from build123d import *

# Parameters (mm, degrees)
F0_R     = 3
F0_R_2   = 18
F0_R_3   = 9
F0_R_4   = 4.5
F1_DEPTH = 5


with BuildPart() as f1:
    # F0 (on Top) → F1 (new body)
    with BuildSketch(Plane.XY):
        Polygon((52.5, 54.183173), (-66, 54.183173), (-66, -68.816827), (-66, -94.316827), (-16.5, -94.316827), (-16.5, -68.816827), (52.5, -68.816827), align=None)
        Polygon((-61.5, -86.816827), (-61.5, -77.816827), (-52.5, -77.816827), (-45, -77.816827), (-36, -77.816827), (-30, -77.816827), (-21, -77.816827), (-21, -86.816827), (-30, -86.816827), (-36, -86.816827), (-45, -86.816827), (-52.5, -86.816827), align=None, mode=Mode.SUBTRACT)
        with Locations((-57, -59.816827)):
            Circle(F0_R, mode=Mode.SUBTRACT)
        with Locations((-33, -32.316827)):
            Circle(F0_R_2, mode=Mode.SUBTRACT)
        with Locations((43.5, -59.816827)):
            Circle(F0_R, mode=Mode.SUBTRACT)
        with Locations((6, -32.316827)):
            Circle(F0_R_3, mode=Mode.SUBTRACT)
        with Locations((31.5, -32.316827)):
            Circle(F0_R_3, mode=Mode.SUBTRACT)
        with Locations((-29.488925, 2.183173)):
            Circle(F0_R, mode=Mode.SUBTRACT)
        with BuildLine():
            Line((-51, 12.183173), (-51, 36.183173))
            Line((-51, 36.183173), (-27, 36.183173))
            ThreePointArc((-27, 36.183173), (-23.25, 32.433173), (-27, 28.683173))
            Line((-27, 28.683173), (-43.5, 28.683173))
            Line((-43.5, 28.683173), (-43.5, 12.183173))
            Line((-43.5, 12.183173), (-51, 12.183173))
        make_face(mode=Mode.SUBTRACT)
        with Locations((-57, 45.183173)):
            Circle(F0_R, mode=Mode.SUBTRACT)
        with BuildLine():
            Line((-6, -1.316827), (-6, 16.683173))
            ThreePointArc((-6, 16.683173), (0, 22.683173), (6, 16.683173))
            Line((6, 16.683173), (6, -1.316827))
            ThreePointArc((6, -1.316827), (0, -7.316827), (-6, -1.316827))
        make_face(mode=Mode.SUBTRACT)
        with Locations((24, 2.183173)):
            Circle(F0_R, mode=Mode.SUBTRACT)
        with Locations((37, 2.183173)):
            Circle(F0_R_4, mode=Mode.SUBTRACT)
        with Locations((43.5, 45.183173)):
            Circle(F0_R, mode=Mode.SUBTRACT)
    extrude(amount=F1_DEPTH)


solid = f1.part
Check sheet for the modelled part. Datum: model origin and axes. Units: mm. A direction names the side the tool comes from. Round coordinates to 2 decimals unless told otherwise and drop trailing zeros. Loops run counter-clockwise (first coordinate to the right, second up) from the corner with the lowest first, then second, coordinate; pieces in that order, holes last. Notation, with made-up numbers: M 52.25,56 L 98.25,56 A31 ccw 98.25,85 Z; hole C 31,29.5 d10. An arc over 180 degrees is marked long. One line per question, with ' | ' between items. Start each with the question number.
Item 1: Gauge pin test, flat end, axial feed: pin 1 Ø7 at (x, y) = (43.5, 45.18) entering from +Z. Record the tip position at first contact, or that the pin passes through.
Item 2: Release check for a two-part mould opening along X. For faces 4 (the face through (4.828, -23.393, 2.465)), 5 (the face through (-8, -19, 0)), 6 (the face through (-66, -19, 2)) record: released by +X, released by -X, zero draft, split by the parting line, or undercut.
Item 3: Section check A-A (y = -80.5). Record the boundary of the cut face in (x, z).
Item 4: Section check C-C (y = -37.5). Record the boundary of the cut face in (x, z).
Item 5: Scan lines: probe 1 along Y at (x, z) = (43.5, 1.8); probe 2 along X at (y, z) = (15.5, 3.5); probe 3 along Y at (x, z) = (31, 2). Record each from-to range of solid material in increasing order.
Item 6: Set-up check for faces 1 (the face through (-16.5, -82, 2)), 2 (the face through (-43.5, 21, 2)), 3 (the face through (-8, -19, 5)): record each of +Z, -Z, +X, -X, +Y, -Y from which the full face is reachable in a straight line by a thin tool's end or side.
Item 7: Section check B-B (x = -57). Record the boundary of the cut face in (y, z).
Item 8: Section check D-D (x = 0). Record the boundary of the cut face in (y, z).
Worked out:
1) pin 1: z = 5
2) face 4: undercut | face 5: zero draft | face 6: released by -X
3) outline: M -66,0 L -61.5,0 L -61.5,5 L -66,5 Z; M -21,0 L -16.5,0 L -16.5,5 L -21,5 Z
4) outline: M -66,0 L -50.24,0 L -50.24,5 L -66,5 Z; M -15.76,0 L -1.36,0 L -1.36,5 L -15.76,5 Z; M 13.36,0 L 24.14,0 L 24.14,5 L 13.36,5 Z; M 38.86,0 L 52.5,0 L 52.5,5 L 38.86,5 Z
5) probe 1: -68.82 to -62.82, -56.82 to 42.18, 48.18 to 54.18 | probe 2: -66 to -51, -43.5 to -6, 6 to 52.5 | probe 3: -68.82 to -41.3, -23.33 to 54.18
6) face 1: +Z, -Z, +X, -Y | face 2: +Z, -Z | face 3: +Z, +X, -X, +Y, -Y
7) outline: M -94.32,0 L -86.82,0 L -86.82,5 L -94.32,5 Z; M -77.82,0 L -62.82,0 L -62.82,5 L -77.82,5 Z; M -56.82,0 L 42.18,0 L 42.18,5 L -56.82,5 Z; M 48.18,0 L 54.18,0 L 54.18,5 L 48.18,5 Z
8) outline: M -68.82,0 L -39.03,0 L -39.03,5 L -68.82,5 Z; M -25.61,0 L -7.32,0 L -7.32,5 L -25.61,5 Z; M 22.68,0 L 54.18,0 L 54.18,5 L 22.68,5 Z
